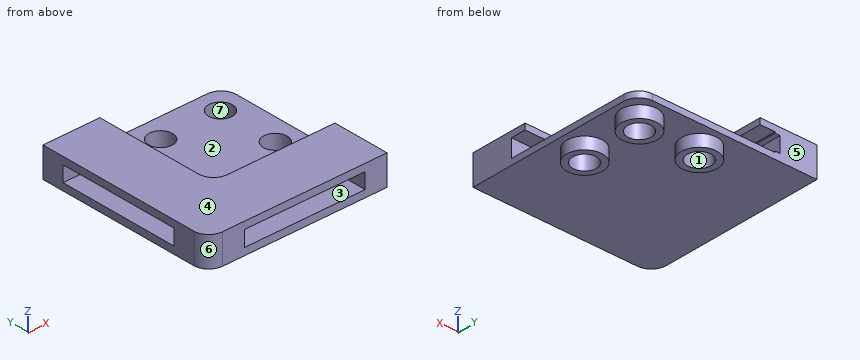
from build123d import *

# Parameters (mm, degrees)
F1_DEPTH  = 1.27
F3_DEPTH  = 3.81
F5_DEPTH  = 1.27
F6_W      = 25.654
F6_H      = 3.302
F7_DEPTH  = 38.101
F8_W      = 25.654
F8_H      = 3.302
F9_DEPTH  = 25.4
F10_R     = 3.81
F11_DEPTH = 2.54
F13_D     = 5.08


with BuildPart() as f1:
    # F0 (on Top) → F1 (new body)
    with BuildSketch(Plane.XY):
        with BuildLine():
            Line((0, 38.1), (0, 3.175))
            ThreePointArc((0, 3.175), (0.929936, 0.929936), (3.175, 0))
            Line((3.175, 0), (38.1, 0))
            Line((38.1, 0), (38.1, 34.925))
            ThreePointArc((38.1, 34.925), (37.170064, 37.170064), (34.925, 38.1))
            Line((34.925, 38.1), (0, 38.1))
        make_face()
    extrude(amount=F1_DEPTH)

    # F2 (on face) → F3 (join)
    with BuildSketch(Plane.XY.offset(1.27)):
        with BuildLine():
            Line((0, 38.1), (0, 3.175))
            ThreePointArc((0, 3.175), (0.929936, 0.929936), (3.175, 0))
            Line((3.175, 0), (38.1, 0))
            Line((38.1, 0), (38.1, 8.89))
            Line((38.1, 8.89), (8.89, 8.89))
            Line((8.89, 8.89), (8.89, 38.1))
            Line((8.89, 38.1), (0, 38.1))
        make_face()
    extrude(amount=F3_DEPTH)

    # F4 (on face) → F5 (join)
    with BuildSketch(Plane.XY.offset(5.08)):
        with BuildLine():
            Line((12.065, 38.1), (8.89, 38.1))
            Line((8.89, 38.1), (0, 38.1))
            Line((0, 38.1), (0, 3.175))
            ThreePointArc((0, 3.175), (0.929936, 0.929936), (3.175, 0))
            Line((3.175, 0), (38.1, 0))
            Line((38.1, 0), (38.1, 8.89))
            Line((38.1, 8.89), (38.1, 12.065))
            Line((38.1, 12.065), (15.24, 12.065))
            ThreePointArc((15.24, 12.065), (12.994936, 12.994936), (12.065, 15.24))
            Line((12.065, 15.24), (12.065, 38.1))
        make_face()
    extrude(amount=F5_DEPTH)

    # F6 (on face) → F7 (cut, through all)
    with BuildSketch(Plane.XZ):
        with Locations((20.6375, 3.175)):
            Rectangle(F6_W, F6_H)
    extrude(amount=-F7_DEPTH, mode=Mode.SUBTRACT)

    # F8 (on face) → F9 (cut)
    with BuildSketch(Plane(origin=(0, 0, 0), x_dir=(0, -1, 0), z_dir=(-1, 0, 0))):
        with Locations((-20.6375, 3.175)):
            Rectangle(F8_W, F8_H)
    extrude(amount=-F9_DEPTH, mode=Mode.SUBTRACT)

    # F10 (on face) → F11 (join)
    with BuildSketch(Plane(origin=(0, 0, 0), x_dir=(1, 0, 0), z_dir=(0, 0, -1))):
        with Locations((33.02, -33.02)):
            Circle(F10_R)
        with Locations((33.02, -20.32)):
            Circle(F10_R)
        with Locations((20.32, -33.02)):
            Circle(F10_R)
    extrude(amount=F11_DEPTH)

    # F13 (through all)
    with Locations(Plane(origin=(0, 0, -2.54), x_dir=(1, 0, 0), z_dir=(0, 0, -1))):
        with Locations((20.32, -33.02), (33.02, -33.02), (33.02, -20.32)):
            Hole(F13_D / 2)


solid = f1.part
Read the model definition and answer for the solid it produces. Units are mm, in the model's axes. Face numbers are marked on the shaded views. A direction names the side the tool comes from. Give positions to 0.01 mm unless a question says otherwise; leave off trailing zeros. Write each loop counter-clockwise with the first axis right and the second up, starting at its lowest first coordinate (ties: lowest second). Pieces come first, ordered by that corner, then holes. Notation, with made-up numbers: (22.25, 37) - (51.25, 37) arc R33 cw to (51.25, 73) - close; hole circle Ø5 at (28.5, 39). An arc over 180 degrees is marked (long way). Answer in a Markdown table with one row per item. Add a question column.
Item 1: Determine the mould class of the marked faces 4, 5, 6 and 7 for opening direction Y: pulls with the +Y half, pulls with the -Y half, needs draft (parallel to the pull), parting line crosses it, or undercut.
Item 2: Section A-A, the plane x = 33.02 is taken. Write down the section's boundary in (y, z) (3 decimals), and give its area (3 significant figures).
Item 3: Section B-B, the plane z = -0.75 is taken. Write down the section's boundary in (x, y).
Item 4: A tool of negligible diameter and unlimited length cuts with its end or side. For the marked faces 1, 2 and 3, from which of +Z, -Z, +X, -X, +Y, -Y can it reach the whole face along a straight path? Write none if from no direction.
Item 5: Flat-ended cylindrical pins translate along their axes: P1, Ø3.5, axis at y = 35.5, z = 2.5, coming from the +X side; P2, Ø1, axis at y = 32.5, z = 5.5, coming from the +X side (3 decimals); P3, Ø4, axis at x = 26, y = 18, coming from the -Z side; P4, Ø6.5, axis at x = 33.02, y = 20.32, coming from the +Z side. Find the tip coordinate at first contact, or state that the pin passes through.
Item 6: Find the intervals of material crossed by L1, parallel to X at y = 33, z = -1.25; L2, parallel to Z at x = 9, y = 25, in increasing order.
Item 7: Section D-D, the plane x = 11.5 is taken. Write down the section's boundary in (y, z), and give its area (3 significant figures).
Recorded:
| question | item | result |
|---|---|---|
| 1 | face 4 | needs draft |
| 1 | face 5 | pulls with the +Y half |
| 1 | face 6 | pulls with the -Y half |
| 1 | face 7 | undercut |
| 2 | outline | (0, 0) - (16.51, 0) - (16.51, -2.54) - (17.78, -2.54) - (17.78, 1.27) - (8.89, 1.27) - (8.89, 1.524) - (0, 1.524) - close; (0, 4.826) - (8.89, 4.826) - (8.89, 5.08) - (12.065, 5.08) - (12.065, 6.35) - (0, 6.35) - close; (22.86, -2.54) - (24.13, -2.54) - (24.13, 0) - (29.21, 0) - (29.21, -2.54) - (30.48, -2.54) - (30.48, 1.27) - (22.86, 1.27) - close; (35.56, -2.54) - (36.83, -2.54) - (36.83, 0) - (38.1, 0) - (38.1, 1.27) - (35.56, 1.27) - close |
| 2 | area | 68.2 mm2 |
| 3 | outline | circle Ø7.62 at (20.32, 33.02); circle Ø7.62 at (33.02, 20.32); circle Ø7.62 at (33.02, 33.02); hole circle Ø5.08 at (20.32, 33.02); hole circle Ø5.08 at (33.02, 20.32); hole circle Ø5.08 at (33.02, 33.02) |
| 4 | face 1 | +Z, -Z |
| 4 | face 2 | +X, +Y |
| 4 | face 3 | none |
| 5 | P1 | stops at x = 38.1 |
| 5 | P2 | stops at x = 12.065 |
| 5 | P3 | stops at z = 0 |
| 5 | P4 | stops at z = 1.27 |
| 6 | L1 | x = 16.51 to 17.78, 22.86 to 24.13, 29.21 to 30.48, 35.56 to 36.83 |
| 6 | L2 | z = 0 to 1.27, 5.08 to 6.35 |
| 7 | outline | (0, 0) - (38.1, 0) - (38.1, 1.27) - (8.89, 1.27) - (8.89, 1.52) - (0, 1.52) - close; (0, 4.83) - (8.89, 4.83) - (8.89, 5.08) - (38.1, 5.08) - (38.1, 6.35) - (0, 6.35) - close |
| 7 | area | 101 mm2 |
